Autodesk Fusion 360 part; units mm, degrees
sketch "Sketch1" plane through (0, 0, 0) normal (0, 1, 0) x (1, 0, 0)
  circle A0 centre (0, 0) radius 10
  circle A1 centre (0, 0) radius 4.5
  circle A2 centre (0, 0) radius 2.75
  circle A3 centre (0, 0) radius 1.5
  dimension "d1" = 20
  dimension "d2" = 9
  dimension "d3" = 5.5
  dimension "d4" = 3
extrude "Extrude1" add sketch "Sketch1" along normal blind 2 contours A0
extrude "Extrude2" add sketch "Sketch1" along normal blind 4.5 contours A1
extrude "Extrude3" add sketch "Sketch1" along normal blind 1 contours A2
sketch "Sketch2" plane through (0, 2, 0) normal (0, 1, 0) x (-1, 0, 0)
  circle A0 centre (0, 0) radius 4.5
  circle A1 centre (0, 0) radius 10
  circle A2 centre (0, 0) radius 7
  line L0 (0, 0) -> (7, 0)
  circle A3 centre (7, 0) radius 1.5
  dimension "d11" = 14
  dimension "d12" = 3
extrude "Extrude4" cut sketch "Sketch2" against normal blind 2 contours A2 L0 A3 | A2 L0 A3 | A2 A3 picked at (7.4507, 0.3705)
pattern_circular "C-Pattern1" count 4 over 360 about axis through (0, 1.75, 0) along (0, 1, 0) of "Extrude4"
thread "Thread1"
thread "Thread2"
thread "Thread3"
thread "Thread4"
sketch "Sketch3" plane through (0, 4.5, 0) normal (0, 1, 0) x (-1, 0, 0)
  circle A0 centre (0, 0) radius 2.75
  circle A1 centre (0, 0) radius 4.5
  circle A2 centre (0, 0) radius 3
  line L0 (0, 0) -> (3, 0)
  line L1 (0, 0) -> (2.9763, -0.376)
  line L2 (0, 0) -> (2.9057, -0.7461)
  line L3 (2.75, 0) -> (2.9763, -0.376)
  line L4 (2.6636, -0.6839) -> (2.9763, -0.376)
  dimension "d18" = 7.2
  dimension "d19" = 7.2
  dimension "d20" = 6
extrude "Extrude5" cut sketch "Sketch3" against normal blind 3.5 contours A0 L1 L3 | A0 L1 L4
pattern_circular "C-Pattern2" count 25 over 360 about axis through (0, 1.75, 0) along (0, 1, 0) of "Extrude5"
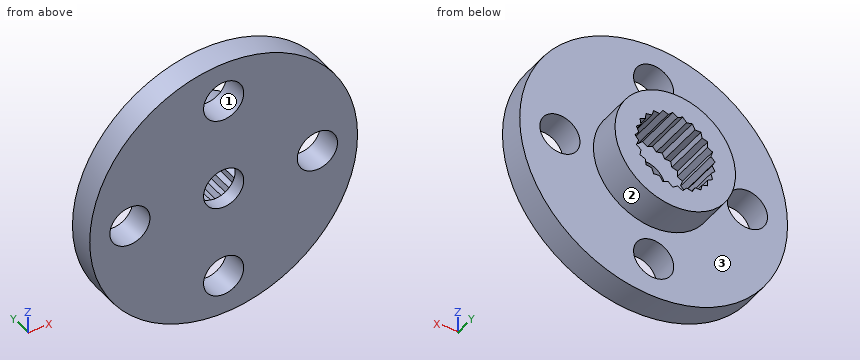
The listing builds one solid part. Answer for the finished solid, in the listing's coordinates (mm). Face numbers are marked on the shaded views. Round coordinates to 2 decimals unless told otherwise and drop trailing zeros. Loops run counter-clockwise (first coordinate to the right, second up) from the corner with the lowest first, then second, coordinate; pieces in that order, holes last. Notation, with made-up numbers: M -21,40 L -15,40 A16 cw -15,45 Z; hole C -6,79 d8. An arc over 180 degrees is marked long. Write each question's results on one line, items separated by ' | '. Start each with the question number.
1) Find section B-B on x = 6.25. Write down the section's boundary in (y, z), plus the area to 3 significant figures.
2) Find section A-A on z = 6. Write down the section's boundary in (x, y).
3) Find section C-C on x = -3.75. Write down the section's boundary in (y, z).
4) Each of these flat-tipped pins is pushed along its axis until it touches: pin 1 (4 mm diameter, centred on x = 0, z = 0, fed in from +Y); pin 2 (1 mm diameter, centred on x = 2.5, z = -4.5, fed in from +Y); pin 3 (1 mm diameter, centred on x = -3, y = 3.5, fed in from +Z); pin 4 (6 mm diameter, centred on x = -4, z = -3, fed in from +Y). Where does it stop, or does it pass through?
5) Determine the mould class of the marked faces 1, 2 and 3 for opening direction Z: pulls with the +Z half, pulls with the -Z half, needs draft (parallel to the pull), parting line crosses it, or undercut.
6) Find section D-D on z = 4. Write down the section's boundary in (x, y).
7) Straight lines are drawn through the part: probe 1 along X at (y, z) = (0.7, 0); probe 2 along Z at (x, y) = (0, 1.15). For each, find the intervals that lie inside material, in ascending order.
Final values:
1) outline: M 0,-7.81 L 2,-7.81 L 2,-1.3 L 0,-1.3 Z; M 0,1.3 L 2,1.3 L 2,7.81 L 0,7.81 Z | area: 26.0 mm²
2) outline: M -8,0 L -1.12,0 L -1.12,2 L -8,2 Z; M 1.12,0 L 8,0 L 8,2 L 1.12,2 Z
3) outline: M 0,-9.27 L 2,-9.27 L 2,-2.49 L 4.5,-2.49 L 4.5,2.49 L 2,2.49 L 2,9.27 L 0,9.27 Z
4) pin 1: y = 1 | pin 2: y = 2 | pin 3: z = 3.74 | pin 4: y = 4.5
5) face 1: undercut | face 2: parting line crosses it | face 3: needs draft
6) outline: M -9.17,0 L 9.17,0 L 9.17,2 L 2.06,2 L 2.06,4.5 L -2.06,4.5 L -2.06,2 L -9.17,2 Z
7) probe 1: -10 to -8.5, -5.5 to -1.5, 1.5 to 5.5, 8.5 to 10 | probe 2: -10 to -8.5, -5.5 to -2.86, 2.86 to 5.5, 8.5 to 10
